```python
from build123d import *

# Parameters (mm, degrees)
SKETCH2_W               = 900
SKETCH2_H               = 51
BOSS_EXTRUDE1_DEPTH     = 1
SKETCH3_W               = 900
SKETCH3_H               = 1
BOSS_EXTRUDE2_DEPTH     = 23.25
BOSS_EXTRUDE3_START     = 1
SKETCH4_W               = 900
SKETCH4_H               = 1
BOSS_EXTRUDE3_DEPTH     = 126
SKETCH5_R               = 2.5
CUT_EXTRUDE1_DEPTH      = 469.272623586
LPATTERN2_COUNT         = 6
LPATTERN2_PITCH         = 200
BOSS_EXTRUDE4_DEPTH     = 127
BOSS_EXTRUDE5_DEPTH     = 127
MIRROR4_COPY_1_SKETCH_R = 2.5
MIRROR4_COPY_1_DEPTH    = 469.272623586
MIRROR4_COPY_2_SKETCH_R = 2.5
MIRROR4_COPY_2_DEPTH    = 469.272623586
MIRROR4_COPY_3_SKETCH_R = 2.5
MIRROR4_COPY_3_DEPTH    = 469.272623586
MIRROR4_COPY_4_SKETCH_R = 2.5
MIRROR4_COPY_4_DEPTH    = 469.272623586
MIRROR4_COPY_5_SKETCH_R = 2.5
MIRROR4_COPY_5_DEPTH    = 469.272623586


with BuildPart() as part:
    # Sketch2 → Boss-Extrude1 (new body)
    with BuildSketch(Plane.XY):
        Rectangle(SKETCH2_W, SKETCH2_H)
    boss_extrude1 = extrude(amount=BOSS_EXTRUDE1_DEPTH)

    # Sketch3 → Boss-Extrude2 (add)
    with BuildSketch(Plane.XY):
        with Locations((0, -25)):
            Rectangle(SKETCH3_W, SKETCH3_H)
    boss_extrude2 = extrude(amount=-BOSS_EXTRUDE2_DEPTH)

    # Sketch4 → Boss-Extrude3 (add)
    with BuildSketch(Plane.XY.offset(BOSS_EXTRUDE3_START)):
        with Locations((0, 25)):
            Rectangle(SKETCH4_W, SKETCH4_H)
    boss_extrude3 = extrude(amount=BOSS_EXTRUDE3_DEPTH)

    # Sketch5 → Cut-Extrude1 (cut, symmetric)
    with BuildSketch(Plane(origin=(0, 0, 0), x_dir=(1, 0, 0), z_dir=(0, 1, 0))):
        with Locations(Location((400, 15, 0), (0, 0, 270))):
            Circle(SKETCH5_R)
    cut_extrude1 = extrude(amount=CUT_EXTRUDE1_DEPTH, both=True, mode=Mode.SUBTRACT)

    # LPattern2: Cut-Extrude1 ×6
    with Locations(*[(-i * LPATTERN2_PITCH, 0, 0) for i in range(1, LPATTERN2_COUNT)]):
        add(cut_extrude1, mode=Mode.SUBTRACT)

    # Sketch7 → Boss-Extrude4 (add)
    with BuildSketch(Plane.XY):
        with BuildLine():
            Line((-450, 24.5), (-450, 25.5))
            ThreePointArc((-450, 25.5), (-453.826834324, 24.738795325), (-457.071067812, 22.571067812))
            Line((-457.071067812, 22.571067812), (-456.363961031, 21.863961031))
            ThreePointArc((-456.363961031, 21.863961031), (-453.444150891, 23.814915793), (-450, 24.5))
        make_face()
    boss_extrude4 = extrude(amount=BOSS_EXTRUDE4_DEPTH)

    # Sketch8 → Boss-Extrude5 (add)
    with BuildSketch(Plane.XY):
        with BuildLine():
            Line((456.363961031, 21.863961031), (457.071067812, 22.571067812))
            ThreePointArc((457.071067812, 22.571067812), (453.826834324, 24.738795325), (450, 25.5))
            Line((450, 25.5), (450, 24.5))
            ThreePointArc((450, 24.5), (453.444150891, 23.814915793), (456.363961031, 21.863961031))
        make_face()
    boss_extrude5 = extrude(amount=BOSS_EXTRUDE5_DEPTH)

    # Mirror2: Boss-Extrude3, Boss-Extrude4, Boss-Extrude5 across plane
    add(boss_extrude3.mirror(Plane.XY.offset(127)))
    add(boss_extrude4.mirror(Plane.XY.offset(127)))
    add(boss_extrude5.mirror(Plane.XY.offset(127)))

    # Mirror4: Boss-Extrude1, Boss-Extrude2, Cut-Extrude1 across plane
    add(boss_extrude1.mirror(Plane.XY.offset(127)))
    add(boss_extrude2.mirror(Plane.XY.offset(127)))
    add(cut_extrude1.mirror(Plane.XY.offset(127)), mode=Mode.SUBTRACT)

    # Mirror4 copy 1 sketch → Mirror4 copy 1 (cut, symmetric)
    with BuildSketch(Plane(origin=(-200, 0, 254), x_dir=(1, 0, 0), z_dir=(0, 1, 0))):
        with Locations((400, -15)):
            Circle(MIRROR4_COPY_1_SKETCH_R)
    extrude(amount=MIRROR4_COPY_1_DEPTH, both=True, mode=Mode.SUBTRACT)

    # Mirror4 copy 2 sketch → Mirror4 copy 2 (cut, symmetric)
    with BuildSketch(Plane(origin=(-400, 0, 254), x_dir=(1, 0, 0), z_dir=(0, 1, 0))):
        with Locations((400, -15)):
            Circle(MIRROR4_COPY_2_SKETCH_R)
    extrude(amount=MIRROR4_COPY_2_DEPTH, both=True, mode=Mode.SUBTRACT)

    # Mirror4 copy 3 sketch → Mirror4 copy 3 (cut, symmetric)
    with BuildSketch(Plane(origin=(-600, 0, 254), x_dir=(1, 0, 0), z_dir=(0, 1, 0))):
        with Locations((400, -15)):
            Circle(MIRROR4_COPY_3_SKETCH_R)
    extrude(amount=MIRROR4_COPY_3_DEPTH, both=True, mode=Mode.SUBTRACT)

    # Mirror4 copy 4 sketch → Mirror4 copy 4 (cut, symmetric)
    with BuildSketch(Plane(origin=(-800, 0, 254), x_dir=(1, 0, 0), z_dir=(0, 1, 0))):
        with Locations((400, -15)):
            Circle(MIRROR4_COPY_4_SKETCH_R)
    extrude(amount=MIRROR4_COPY_4_DEPTH, both=True, mode=Mode.SUBTRACT)

    # Mirror4 copy 5 sketch → Mirror4 copy 5 (cut, symmetric)
    with BuildSketch(Plane(origin=(-1000, 0, 254), x_dir=(1, 0, 0), z_dir=(0, 1, 0))):
        with Locations((400, -15)):
            Circle(MIRROR4_COPY_5_SKETCH_R)
    extrude(amount=MIRROR4_COPY_5_DEPTH, both=True, mode=Mode.SUBTRACT)


solid = part.part
```
Can you work these out from the model? Positions are in its coordinate system, mm. A direction names the side the tool comes from. Coordinates: 2 decimals unless noted, no trailing zeros. Loops run counter-clockwise (first coordinate to the right, second up) from the corner with the lowest first, then second, coordinate; pieces in that order, holes last. Notation, with made-up numbers: M 47,78.5 L 60,78.5 A25 cw 60,94.5 Z; hole C 27,-34 d5. An arc over 180 degrees is marked long. Put each result on its own line as item: value. Start each with the question number.
(1) Imagine slicing it at B-B on x = -47. List the corners of the cut face in (y, z) for me, and give its area (4 significant figures).
(2) I need wall thicknesses on probe 1 along X at (y, z) = (-25.05, 269); probe 2 along Z at (x, y) = (400, -25); probe 3 along Z at (x, y) = (400, -24). Which ranges of each line are inside material? Lowest first, please.
(3) Imagine slicing it at A-A on y = 12.5. List the corners of the cut face in (x, z) for me.
(4) Imagine slicing it at C-C on z = 95. List the corners of the cut face in (x, y) for me, and give its area (3 significant figures).
(5) We'd pull the mould along Z, two halves only. Please class faces 4 (the face through (-6, -24.5, 265)), 5 (the face through (-6, 1, 254)), 6 (the face through (-6, 0, 253)): +Z half, -Z half, draft (parallel to the pull), parting line (faces both ways), or undercut.
(6) Will these pins go through, and if not, where does the flat tip stop? pin 1 Ø5 at (x, y) = (55, -4) entering from -Z; pin 2 Ø1 at (x, z) = (-158, 178) entering from -Y; pin 3 Ø6.5 at (x, z) = (-200, 269) entering from +Y.
(7) Which directions (+Z, -Z, +X, -X, +Y, -Y) give clear straight access to the entire face, cutting with the end or side of a thin tool? Please do faces 1 (the face through (-6, 1, 0)), 2 (the face through (-6, 24.5, 129)), 3 (the face through (-6, -25.5, -11)).
Worked answers:
1. outline: M -25.5,-23.25 L -24.5,-23.25 L -24.5,0 L 25.5,0 L 25.5,254 L -24.5,254 L -24.5,277.25 L -25.5,277.25 L -25.5,253 L 24.5,253 L 24.5,1 L -25.5,1 Z
1. area: 400.5 mm2
2. probe 1: x = -450 to -402.5, -397.5 to -202.5, -197.5 to -2.5, 2.5 to 197.5, 202.5 to 397.5, 402.5 to 450
2. probe 2: z = -23.25 to -17.5, -12.5 to 1, 253 to 266.5, 271.5 to 277.25
2. probe 3: z = 0 to 1, 253 to 254
3. outline: M -450,0 L 450,0 L 450,1 L -450,1 Z; M -450,253 L 450,253 L 450,254 L -450,254 Z
4. outline: M -457.07,22.57 L -456.36,21.86 A9 cw -450,24.5 L 450,24.5 A9 cw 456.36,21.86 L 457.07,22.57 A10 ccw 450,25.5 L -450,25.5 A10 ccw Z
4. area: 915 mm2
5. face 4: draft
5. face 5: +Z half
5. face 6: undercut
6. pin 1: stops at z = 0
6. pin 2: stops at y = 24.5
6. pin 3: stops at y = -24.5
7. face 1: -Z, +X, -X, +Y
7. face 2: -Y
7. face 3: +Z, -Z, +X, -X, -Y
